Autodesk Inventor part; units mm, degrees
ref_plane "Start Plane" through (0, 0, 0) normal (0, 0, 1) x (1, 0, 0)
ref_plane "End Plane" through (0, 0, 2000) normal (0, 0, 1) x (1, 0, 0)
ref_plane "YZ Plane" through (0, 0, 0) normal (1, 0, 0) x (0, 1, 0)
ref_plane "Start Plane" through (0, 0, 0) normal (0, 0, 1) x (1, 0, 0)
ref_plane "End Plane" through (0, 0, 2000) normal (0, 0, 1) x (1, 0, 0)
sketch "Sketch" plane through (0, 0, 0) normal (0, 0, 1) x (1, 0, 0)
  line L0 (-40, -34) -> (-40, 34)
  line L1 (-34, 40) -> (34, 40)
  line L2 (40, 34) -> (40, -34)
  line L3 (34, -40) -> (-34, -40)
  arc A0 (-40, -34) -> (-34, -40) centre (-34, -34) ccw
  arc A1 (40, 34) -> (34, 40) centre (34, 34) ccw
  arc A2 (-34, 40) -> (-40, 34) centre (-34, 34) ccw
  arc A3 (34, -40) -> (40, -34) centre (34, -34) ccw
  arc A4 (-34, 37) -> (-37, 34) centre (-34, 34) ccw
  line L4 (-34, 37) -> (34, 37)
  arc A5 (37, 34) -> (34, 37) centre (34, 34) ccw
  line L5 (37, 34) -> (37, -34)
  arc A6 (34, -37) -> (37, -34) centre (34, -34) ccw
  line L6 (34, -37) -> (-34, -37)
  arc A7 (-37, -34) -> (-34, -37) centre (-34, -34) ccw
  line L7 (-37, -34) -> (-37, 34)
  line L8 (0, 57.7397) -> (0, -57.7397) construction
  line L9 (-57.7397, 0) -> (57.7397, 0) construction
  dimension "d7" = 6
  dimension "d9" = 80
  dimension "d11" = 80
  dimension "d12" = 3
  dimension "d15" = 40
  dimension "d16" = 40
extrude "Body" add sketch "Sketch" along normal up to surface (2000 mm away) from surface at 0
sketch "Sketch3" plane through (0, 0, 0) normal (0, 0, 1) x (1, 0, 0)
  line L0 (0, 0) -> (10, 0)
ref_plane "Work Plane3" through (0, 0, 0) normal (0, -1, 0) x (1, 0, 0)
sketch "Sketch5" plane through (0, 0, 0) normal (0, 1, 0) x (-1, 0, 0)
  line L0 (40, 0) -> (40, 2000)
  line L1 (34, 0) -> (40, 0)
  line L2 (34, 0) -> (-34, 0)
  line L3 (-40, 0) -> (-34, 0)
  line L4 (-40, 0) -> (-40, 2000)
  line L5 (-40, 2000) -> (-34, 2000)
  line L6 (34, 2000) -> (-34, 2000)
  line L7 (34, 2000) -> (40, 2000)
  line L8 (-40, 0) -> (40, 80)
  line L9 (-40, 2000) -> (40, 1920)
  point P0 (0, 0)
  dimension "d19" = 45
  dimension "d20" = 45
extrude "Extrusion2" cut sketch "Sketch5" along normal through all both and the other way through all contours L1 L2 L3 L8 L0 | L9 L5 L6 L7 L0
sketch "Sketch4" plane through (0, 0, 0) normal (0, -1, 0) x (1, 0, 0)
  line L0 (-2, 0) -> (12, 0)
  line L1 (-2, 2000) -> (12, 2000)
  dimension "d18" = 2000
equation "\"d7\" = G_IR"
equation "\"d9\" = G_W"
equation "\"d11\" = G_H"
equation "\"d12\" = G_T"
equation "\"d15\" = 0.5 * d9"
equation "\"d16\" = 0.5 * d11"
equation "\"d3\" = G_L"
equation "\"d20\" = d19"
equation "\"G_W\" = 80"
equation "\"G_H\" = 80"
equation "\"G_T\" = 3"
equation "\"G_IR\" = 6"
equation "\"G_L\" = d18"
equation "\"G_OFFSET_START\" = 0"
equation "\"G_OFFSET_END\" = 0"
properties part number "ISO 4019 - 80x80x3 - 2000" material "Steel, Mild"
Input: part model. Units: mm. Frame: model coordinates. A direction names the side the tool comes from. Give positions to 0.01 mm unless a question says otherwise; leave off trailing zeros. Order: outer loops, then holes, each group sorted by start corner. A loop starts at its lowest first (then second) coordinate and runs counter-clockwise, first axis right, second up.
Q1. Ray query, probe 1 along X at (y, z) = (5, 1185.5). Return the intervals inside material, ascending.
Checked values:
probe 1: x = -40 to -37, 37 to 40
Q2. Section C-C on z = 1831. Output: boundary loops of the cut face in (x, y).
Checked values:
outline: (-40, -34) arc R6 ccw to (-34, -40) - (34, -40) arc R6 ccw to (40, -34) - (40, 34) arc R6 ccw to (34, 40) - (-34, 40) arc R6 ccw to (-40, 34) - close; hole (-37, -34) arc R3 ccw to (-34, -37) - (34, -37) arc R3 ccw to (37, -34) - (37, 34) arc R3 ccw to (34, 37) - (-34, 37) arc R3 ccw to (-37, 34) - close
Q3. Section A-A on y = 20.5. Output: boundary loops of the cut face in (x, z), and give its area (3 significant figures).
Checked values:
outline: (-40, 80) - (-37, 77) - (-37, 1923) - (-40, 1920) - close; (37, 3) - (40, 0) - (40, 2000) - (37, 1997) - close
area: 11,500 mm2
Q4. Draft query along X for faces 3 (the flat face through (0, -39, 40)), 4 (the flat face through (-37, 0, 987)), 5 (the flat face through (40, 0, 986)), 6 (the flat face through (0, 40, 986)). Return one class per face: +X half, -X half, draft (parallel to the pull), parting line (faces both ways), or undercut.
Checked values:
face 3: -X half
face 4: undercut
face 5: +X half
face 6: draft
Q5. Section B-B on x = 19. Output: boundary loops of the cut face in (y, z), and give its area (3 significant figures).
Checked values:
outline: (-40, 21) - (-37, 21) - (-37, 1979) - (-40, 1979) - close; (37, 21) - (40, 21) - (40, 1979) - (37, 1979) - close
area: 11,700 mm2
Q6. Set-up query: faces 1 (the flat face through (-40, 0, 987)), 2 (the flat face through (37, 0, 986)). Return all of +Z, -Z, +X, -X, +Y, -Y with unobstructed straight access to the full face (end or side cutting, diameter ignored); none if empty.
Checked values:
face 1: +Z, -Z, -X, +Y, -Y
face 2: +Z, -Z
